Check sheet for the modelled part. Datum: model origin and axes. Units: mm. A direction names the side the tool comes from. Coordinates: 2 decimals unless noted, no trailing zeros. Loops run counter-clockwise (first coordinate to the right, second up) from the corner with the lowest first, then second, coordinate; pieces in that order, holes last. Notation, with made-up numbers: (9, -13) -> (35, -13) arc R20 ccw to (35, 11) -> close; hole circle Ø3 at (38.5, 16.25). An arc over 180 degrees is marked (long way). Use CSV: the item, a comma, the result in double quotes.
```python
from build123d import *

# Parameters (mm, degrees)
F0_R     = 2.75
F0_W     = 100
F0_H     = 42.47
F1_DEPTH = 4
F2_R     = 2.75
F3_DEPTH = 8
F4_R     = 2.75
F5_DEPTH = 4
F7_R     = 4.125
F8_DEPTH = 18.001


with BuildPart() as f1:
    # F0 (on Top) → F1 (new body)
    with BuildSketch(Plane.XY):
        with BuildLine():
            ThreePointArc((70, 25), (67.0710678119, 32.0710678119), (60, 35))
            Line((60, 35), (-60, 35))
            ThreePointArc((-60, 35), (-67.0710678119, 32.0710678119), (-70, 25))
            Line((-70, 25), (-70, -25))
            ThreePointArc((-70, -25), (-67.0710678119, -32.0710678119), (-60, -35))
            Line((-60, -35), (60, -35))
            ThreePointArc((60, -35), (67.0710678119, -32.0710678119), (70, -25))
            Line((70, -25), (70, 25))
        make_face()
        with Locations((-60, -25)):
            Circle(F0_R, mode=Mode.SUBTRACT)
        with Locations((60, -25)):
            Circle(F0_R, mode=Mode.SUBTRACT)
        with Locations((-60, 25)):
            Circle(F0_R, mode=Mode.SUBTRACT)
        Rectangle(F0_W, F0_H, mode=Mode.SUBTRACT)
        with Locations((60, 25)):
            Circle(F0_R, mode=Mode.SUBTRACT)
    extrude(amount=F1_DEPTH)

    # F2 (on face) → F3 (join)
    with BuildSketch(Plane.YZ.offset(-50)):
        with BuildLine():
            ThreePointArc((-17.3240695981, 7.1605815157), (-18.7208076781, 4.8889170746), (-21.235, 4))
            Line((-21.235, 4), (21.235, 4))
            ThreePointArc((21.235, 4), (18.7208076781, 4.8889170746), (17.3240695981, 7.1605815157))
            Line((17.3240695981, 7.1605815157), (15.6759304019, 14.8394184843))
            ThreePointArc((15.6759304019, 14.8394184843), (14.2791923219, 17.1110829254), (11.765, 18))
            Line((11.765, 18), (-11.765, 18))
            ThreePointArc((-11.765, 18), (-14.2791923219, 17.1110829254), (-15.6759304019, 14.8394184843))
            Line((-15.6759304019, 14.8394184843), (-17.3240695981, 7.1605815157))
        make_face()
        with Locations((-10.11, 11)):
            Circle(F2_R, mode=Mode.SUBTRACT)
        with Locations((10.11, 11)):
            Circle(F2_R, mode=Mode.SUBTRACT)
    extrude(amount=-F3_DEPTH)

    # F4 (on face) → F5 (cut)
    with BuildSketch(Plane(origin=(-58, 0, 0), x_dir=(0, -1, 0), z_dir=(-1, 0, 0))):
        Polygon((-5.2025227119, 11), (-7.6562613559, 15.25), (-12.5637386441, 15.25), (-15.0174772881, 11), (-12.5637386441, 6.75), (-7.6562613559, 6.75), align=None)
        with Locations((-10.11, 11)):
            Circle(F4_R, mode=Mode.SUBTRACT)
        Polygon((7.6562613559, 6.75), (12.5637386441, 6.75), (15.0174772881, 11), (12.5637386441, 15.25), (7.6562613559, 15.25), (5.2025227119, 11), align=None)
        with Locations((10.11, 11)):
            Circle(F4_R, mode=Mode.SUBTRACT)
    extrude(amount=-F5_DEPTH, mode=Mode.SUBTRACT)

    # F6: F1 across plane


with BuildPart() as f1_1:
    add(f1.part)
    add(f1.part.mirror(Plane.YZ))

    # F7 (on face) → F8 (cut, through all)
    with BuildSketch(Plane(origin=(0, 0, 0), x_dir=(1, 0, 0), z_dir=(0, 0, -1))):
        with Locations((-50, 0)):
            Circle(F7_R)
        with Locations((50, 0)):
            Circle(F7_R)
    extrude(amount=-F8_DEPTH, mode=Mode.SUBTRACT)


solid = f1_1.part
```
1) Access from +Z, -Z, +X, -X, +Y, -Y to the whole of each face (thin tool, end or side, straight path). Record for faces 4 (the flat face through (56, 10, 6.75)), 5 (the flat face through (-1, -21.235, 2)), 6 (the flat face through (-56.028, 13.808, 8.905)).
Answer below:
face 4,"+X"
face 5,"+Z, -Z"
face 6,"-X"
2) Cross-section at A-A on y = 0. Record the boundary of the cut face in (x, z) (3 decimals).
Answer below:
outline,"(-70, 0) -> (-54.125, 0) -> (-54.125, 18) -> (-58, 18) -> (-58, 4) -> (-70, 4) -> close; (54.125, 0) -> (70, 0) -> (70, 4) -> (58, 4) -> (58, 18) -> (54.125, 18) -> close"
3) Draft check along Y on faces 1 (the cylindrical face through (53.944, 14.309, 17.087)), 2 (the flat face through (-1, -35, 2)), 3 (the flat face through (56, -10, 15.25)). Enter one of: released by +Y, released by -Y, zero draft, split by the parting line, or undercut.
Answer below:
face 1,"released by +Y"
face 2,"released by -Y"
face 3,"undercut"
4) Thickness scan on line 1 along Y through (x, z) = (-60, 3); line 2 along X through (y, z) = (25, 1.85); line 3 along X through (y, z) = (20.5, 3.5). Record the ranges inside material, lowest first. Write a range as from..to.
Answer below:
line 1,"y = -35..-27.75, -22.25..22.25, 27.75..35"
line 2,"x = -70..-62.75, -57.25..57.25, 62.75..70"
line 3,"x = -70..-50, 50..70"
5) Cross-section at B-B on x = -41.5. Record the boundary of the cut face in (y, z) (3 decimals).
Answer below:
outline,"(-35, 0) -> (-21.235, 0) -> (-21.235, 4) -> (-35, 4) -> close; (21.235, 0) -> (35, 0) -> (35, 4) -> (21.235, 4) -> close"
6) Go/stop test with flat-tipped pins: pin 1 Ø3 at (y, z) = (-18, 8.5) entering from +X; pin 2 Ø4.5 at (x, y) = (-55.5, 9.5) entering from -Z; pin 3 Ø1.5 at (x, z) = (-48.5, 14.5) entering from +Y; pin 4 Ø5 at (y, z) = (15.5, 14) entering from -X. Record where each tip stops, or that it passes through.
Answer below:
pin 1,"stops at x = 58"
pin 2,"stops at z = 0"
pin 3,"passes through"
pin 4,"stops at x = -58"
